For this review, take the finished solid that the model builds, in its own axes (mm). Face numbers are marked on the shaded views. A direction names the side the tool comes from. Coordinates: 2 decimals unless noted, no trailing zeros. Order: outer loops, then holes, each group sorted by start corner. A loop starts at its lowest first (then second) coordinate and runs counter-clockwise, first axis right, second up.
from build123d import *

# Parameters (mm, degrees)
BOSS_EXTRUDE1_DEPTH = 10
SKETCH3_R           = 1.25
CUT_EXTRUDE1_DEPTH  = 10
BOSS_EXTRUDE2_DEPTH = 1


with BuildPart() as part:
    # Sketch2 → Boss-Extrude1 (new body)
    with BuildSketch(Plane(origin=(0, 0, 0), x_dir=(1, 0, 0), z_dir=(0, 1, 0))):
        Polygon((0, 2.5), (-5, 2.5), (-5, -2.5), (-5, -7.5), (-2.5, -7.5), (-2.5, 0), (5, 0), (5, 2.5), align=None)
    extrude(amount=BOSS_EXTRUDE1_DEPTH)

    # Sketch3 → Cut-Extrude1 (cut)
    with BuildSketch(Plane.XY):
        with Locations((1.25, 7)):
            Circle(SKETCH3_R)
    cut_extrude1 = extrude(amount=-CUT_EXTRUDE1_DEPTH, mode=Mode.SUBTRACT)

    # Mirror1: Cut-Extrude1 across plane
    add(cut_extrude1.mirror(Plane(origin=(0, 5, 0), x_dir=(0, 0, 1), z_dir=(0, -1, 0))), mode=Mode.SUBTRACT)

    # Sketch4 → Boss-Extrude2 (add)
    with BuildSketch(Plane(origin=(0, 10, 0), x_dir=(1, 0, 0), z_dir=(0, 1, 0))):
        Polygon((-2.5, -7.5), (5, 0), (-2.5, 0), align=None)
    boss_extrude2 = extrude(amount=-BOSS_EXTRUDE2_DEPTH)

    # Mirror2: Boss-Extrude2 across plane
    add(boss_extrude2.mirror(Plane(origin=(0, 5, 0), x_dir=(0, 0, 1), z_dir=(0, -1, 0))))


solid = part.part
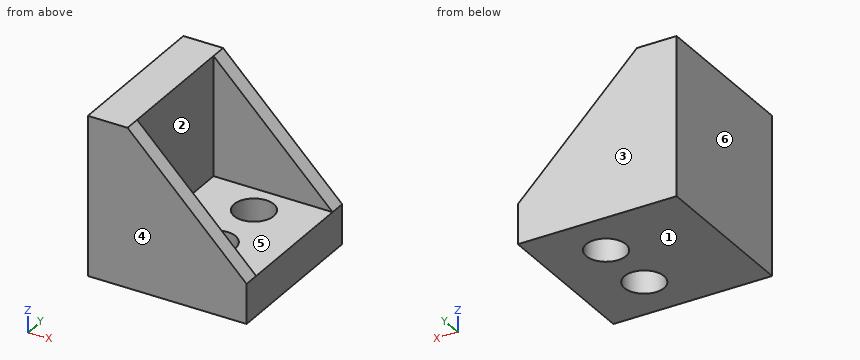
1. Take a section at A-A, the plane x = 1.25. Give the boundary of the cut face in (y, z), plus the area to 3 significant figures.
Answer below:
outline: (0, -2.5) - (1.75, -2.5) - (1.75, 0) - (1, 0) - (1, 3.75) - (0, 3.75) - close; (4.25, -2.5) - (5.75, -2.5) - (5.75, 0) - (4.25, 0) - close; (8.25, -2.5) - (10, -2.5) - (10, 3.75) - (9, 3.75) - (9, 0) - (8.25, 0) - close
area: 20.0 mm2
2. The part is to be moulded in two halves that separate along Y. For the marked faces 1, 2, 3 and 4, say which applies: +Y half, -Y half, draft (parallel to the pull), parting line (faces both ways), or undercut.
Answer below:
face 1: draft
face 2: undercut
face 3: +Y half
face 4: -Y half
3. Take a section at B-B, the plane y = 7. Give the boundary of the cut face in (x, z).
Answer below:
outline: (-5, -2.5) - (0, -2.5) - (0, 0) - (-2.5, 0) - (-2.5, 7.5) - (-5, 7.5) - close; (2.5, -2.5) - (5, -2.5) - (5, 0) - (2.5, 0) - close
4. Take a section at D-D, the plane x = -1. Give the boundary of the cut face in (y, z).
Answer below:
outline: (0, -2.5) - (10, -2.5) - (10, 6) - (9, 6) - (9, 0) - (1, 0) - (1, 6) - (0, 6) - close
5. Machinability: for the marked faces 5 and 6, which of the approach directions +Z, -Z, +X, -X, +Y, -Y give a long, thin tool a straight path to every point of the face, cutting with its end or side? Answer none if there is none.
Answer below:
face 5: +Z, +X
face 6: +Z, -Z, -X, +Y, -Y
6. Clearance check with flat-ended pins moving along their axes: pin 1 Ø2 at (x, y) = (1.25, 3) entering from +Z; pin 2 Ø4 at (x, y) = (1, 4) entering from +Z; pin 3 Ø6 at (x, y) = (-1.5, 5.5) entering from +Z; pin 4 Ø4 at (y, z) = (6.5, 3) entering from +X. State where each tip first meets the part, or that it passes through.
Answer below:
pin 1: passes through
pin 2: stops at z = 0
pin 3: stops at z = 7.5
pin 4: stops at x = -2.5
7. To check wall thickness, follow L1, parallel to Y at x = 1.25, z = -1.05; L2, parallel to Y at x = -1, z = 2; L3, parallel to Z at x = 3.5, y = 5.25. State the ranges of each line that lie inside material, in increasing order.
Answer below:
L1: y = 0 to 1.75, 4.25 to 5.75, 8.25 to 10
L2: y = 0 to 1, 9 to 10
L3: z = -2.5 to 0
8. Take a section at C-C, the plane z = 6.75. Give the boundary of the cut face in (x, y).
Answer below:
outline: (-5, 0) - (-1.75, 0) - (-1.75, 1) - (-2.5, 1) - (-2.5, 9) - (-1.75, 9) - (-1.75, 10) - (-5, 10) - close
